Autodesk Inventor part; units mm, degrees
ref_plane "Work Plane1" through (1.525, 0, 0) normal (0, 0, 1) x (1, 0, 0)
ref_plane "YZ Plane" through (0, 0, 0) normal (1, 0, 0) x (0, 1, 0)
ref_plane "XZ Plane" through (0, 0, 0) normal (0, 1, 0) x (-1, 0, 0)
sketch "Sketch1" plane through (0, 0, 0) normal (0, 0, 1) x (1, 0, 0)
  line L0 (0, 7.7) -> (0, 5)
  line L1 (3, 5) -> (110, 5)
  line L2 (110, 5) -> (110, 0)
  line L3 (110, 0) -> (-0.6001, 0)
  line L4 (-22.7201, 0) -> (132.12, 0)
  line L5 (-0.6001, 0) -> (-0.6001, 7.7)
  line L6 (-0.6001, 7.7) -> (0, 7.7)
  line L7 (3, 5) -> (2.3864, 5)
  line L8 (2.3864, 5) -> (0, 5)
  line L9 (0, -1.54) -> (0, 9.24)
  dimension "d0" = 110
  dimension "d1" = 107
  dimension "d2" = 10
  dimension "d9" = 0.6001
  dimension "d10" = 15.4
  dimension "d13" = 0.6136
  dimension "d14" = 10
revolve "Body" add sketch "Sketch1" angle 360 about axis through (110, 0, 0) along (-1, 0, 0)
sketch "Sketch2" plane through (-0.6001, 0, 0) normal (-1, 0, 0) x (0, 0, 1)
  line L0 (0, 9.815) -> (8.5, 4.9075)
  line L1 (8.5, 4.9075) -> (8.5, -4.9075)
  line L2 (8.5, -4.9075) -> (0, -9.815)
  line L3 (0, -9.815) -> (-8.5, -4.9075)
  line L4 (-8.5, -4.9075) -> (-8.5, 4.9075)
  line L5 (-8.5, 4.9075) -> (0, 9.815)
  point P0 (0, 0)
  point P1 (0, 0)
  dimension "d11" = 17
extrude "Head" add sketch "Sketch2" along normal blind 5.8
sketch "Sketch4" plane through (0, 0, 0) normal (0, 0, 1) x (1, 0, 0)
  line L0 (-6.4001, 8.5) -> (-6.4001, 9.815)
  line L1 (-6.4001, 9.815) -> (-5.6409, 9.815)
  line L2 (-5.6409, 9.815) -> (-6.4001, 8.5)
  line L3 (-7.5601, 0) -> (0.5599, 0)
  line L4 (-0.6001, 9.815) -> (-6.4001, 9.815)
  line L5 (-6.4001, 4.9075) -> (-6.4001, 9.815)
  dimension "d5" = 30
  dimension "d19" = 17
revolve "Chamfer1" cut sketch "Sketch4" angle 360 about axis through (-10, 0, 0) along (1, 0, 0)
thread "Thread"
chamfer "Chamfer2" distance 0.6134 distance2 0.6136 1 edges at (110, -5, 0) measured on face at (110, 0.591, 1.1849)
ref_plane "Work Plane1" through (1.525, 0, 0) normal (0, 0, 1) x (1, 0, 0)
equation "\"d0\" = NLG"
equation "\"d1\" = GEL"
equation "\"d2\" = GD"
equation "\"d10\" = SD2"
equation "\"d14\" = BDM"
equation "\"d11\" = SW"
equation "\"d3\" = KOH - SD"
equation "\"d5\" = ANG1"
equation "\"d19\" = SW0"
equation "\"d15\" = GEL"
equation "\"d6\" = -0.5 * SPD + 0.5 * GD"
equation "\"NLG\" = 110"
equation "\"GD\" = NND"
equation "\"BDM\" = NND"
equation "\"KOH\" = 6.4"
equation "\"GEL\" = 107"
equation "\"SW\" = 17"
equation "\"SW0\" = 17"
equation "\"SPD\" = NND - 1.2269 * PTC"
equation "\"SD2\" = 15.4"
equation "\"SD\" = 0.6"
equation "\"ANG1\" = 30deg"
equation "\"GAL\" = 0.61345 * PTC"
equation "\"GUL\" = 0.61345 * PTC"
equation "\"RR\" = 0"
equation "\"GD1\" = THREADDIA - 1.2269 * PTC"
equation "\"TOA\" = 30deg"
equation "\"FAWI\" = 45deg"
equation "\"PTC\" = 1"
equation "\"E0\" = 1.155 * SW"
properties part number "DIN 961 - M10 x 110" material "Steel, Mild"
The model under review builds one solid part; all positions refer to its coordinate system, in mm. A direction names the side the tool comes from. Round coordinates to 2 decimals unless told otherwise and drop trailing zeros. Write each loop counter-clockwise with the first axis right and the second up, starting at its lowest first coordinate (ties: lowest second). Pieces come first, ordered by that corner, then holes. Notation, with made-up numbers: (-22, 64) - (23, 64) arc R25 ccw to (23, 80) - close; hole circle Ø1 at (-5.5, 44). An arc over 180 degrees is marked (long way). One line per question, with ' | ' between items.
Item 1: Add section A-A, the plane x = 17. Give the boundary of the cut face in (y, z).
Resolved:
outline: circle Ø10 at (0, 0)
Item 2: To check wall thickness, follow probe 1 along Y at (x, z) = (87, 0); probe 2 along X at (y, z) = (-2.25, 7.25); probe 3 along X at (y, z) = (-8, 1.5). State the ranges of each line that lie inside material, in increasing order.
Resolved:
probe 1: y = -5 to 5 | probe 2: x = -6.4 to 0 | probe 3: x = -6.4 to -0.6
Item 3: For faces 1 (the face through (53.93, -1.08, 4.88)), 2 (the face through (110, 0, 0)), list the 3-axis set-ups (+Z, -Z, +X, -X, +Y, -Y) from which the entire face can be reached by the end or side of a thin tool; tool diameter is ignored.
Resolved:
face 1: +X | face 2: +Z, -Z, +X, +Y, -Y
Item 4: For P1, Ø6, axis at x = 43.5, z = 6, coming from the -Y side; P2, Ø6, axis at x = 68, z = -1, coming from the -Y side; P3, Ø3, axis at x = 56, y = -6, coming from the +Z side; P4, Ø1, axis at y = -7.5, z = 5.5, coming from the +X side, all flat-tipped, find the tip position at first contact; note any pin that passes through.
Resolved:
P1: stops at y = -4 | P2: stops at y = -5 | P3: stops at z = 2.18 | P4: passes through
